Autodesk Inventor part; units mm, degrees
ref_plane "YZ Plane" through (0, 0, 0) normal (1, 0, 0) x (0, 1, 0)
ref_plane "XZ Plane" through (0, 0, 0) normal (0, 1, 0) x (-1, 0, 0)
ref_plane "XY Plane" through (0, 0, 0) normal (0, 0, 1) x (1, 0, 0)
sketch "Sketch1" plane through (0, 0, 0) normal (0, 1, 0) x (-1, 0, 0)
  line L0 (0, 0) -> (20, 0)
  line L1 (0, 0) -> (0, -7.35)
  line L2 (0, -7.35) -> (20, -7.35)
  circle A0 centre (28, -3.675) radius 3
  line L3 (20, -7.35) -> (28, -6.675)
  line L4 (20, 0) -> (28, -0.675)
  dimension "d0" = 20
  dimension "d1" = 7.35
extrude "Extrusion1" add sketch "Sketch1" along normal blind 2
sketch "Sketch3" plane through (0, 2, 0) normal (0, 1, 0) x (1, 0, 0)
  line L0 (0, 0) -> (0, 7.35)
  line L1 (-4.5, 2.25) -> (-14, 2.25)
  line L2 (0, 0) -> (0, 3.68)
  line L3 (0, 0) -> (0, 5.1)
  line L4 (-4.5, 5.1) -> (-14, 5.1)
  line L5 (0, 7.35) -> (-20, 7.35)
  line L6 (-20, 0) -> (0, 0)
  arc A0 (-14, 5.1) -> (-14, 2.25) centre (-14, 3.675) ccw
  arc A1 (-4.5, 2.25) -> (-4.5, 5.1) centre (-4.525, 3.675) ccw
extrude "Extrusion3" cut sketch "Sketch3" against normal blind 10
sketch "Sketch4" plane through (0, 2, 0) normal (0, 1, 0) x (1, 0, 0)
  line L0 (0, 0) -> (-28, 0)
  line L1 (-20, 0) -> (0, 0)
  arc A0 (-28, 6.675) -> (-28, 0.675) centre (-28, 3.675) ccw
  line L2 (-28, 0) -> (-28, 6.675)
  dimension "d20" = 28
extrude "Extrusion4" cut sketch "Sketch4" against normal blind 10
sketch "Sketch5" plane through (0, 2, 0) normal (0, 1, 0) x (1, 0, 0)
  line L0 (-28, 0.675) -> (-20, 0)
  line L1 (-20, 0) -> (-20, 7.35)
  line L2 (-20, 7.35) -> (-28, 6.675)
  line L3 (-20, 7.35) -> (-28, 6.675)
  line L4 (-28, 6.675) -> (-28, 0.675)
  line L5 (-28, 0.675) -> (-20, 0)
  point P0 (0, 0)
extrude "Extrusion5" cut sketch "Sketch5" against normal blind 10
sketch "Sketch7" plane through (0, 2, 0) normal (0, 1, 0) x (1, 0, 0)
  line L0 (0, 0) -> (0, 3.675)
  circle A0 centre (-28.5, 3.675) radius 2.5
  line L1 (-20, 0) -> (0, 0)
  line L2 (-20, 0) -> (-28.8358, 1.1977)
  line L3 (0, 7.35) -> (-20, 7.35)
  line L4 (-20, 7.35) -> (-28.8358, 6.1523)
  line L5 (-20, 7.35) -> (-20, 0)
  line L6 (-20, 7.35) -> (-20, 0)
  dimension "d42" = 5
extrude "Extrusion6" add sketch "Sketch7" against normal blind 2
sketch "Sketch8" plane through (0, 2, 0) normal (0, 1, 0) x (1, 0, 0)
  line L0 (0, 0) -> (0, 7.35)
  circle A0 centre (-22, 3.675) radius 0.67
  circle A1 centre (-25, 3.675) radius 0.67
  circle A2 centre (-28, 3.675) radius 0.67
  dimension "d46" = 1.34
  dimension "d48" = 1.34
  dimension "d50" = 1.34
extrude "Extrusion7" cut sketch "Sketch8" against normal blind 2
properties part number "MMAE 232 Assignment 2_Servo Horn 1 - Dylan Tamras"
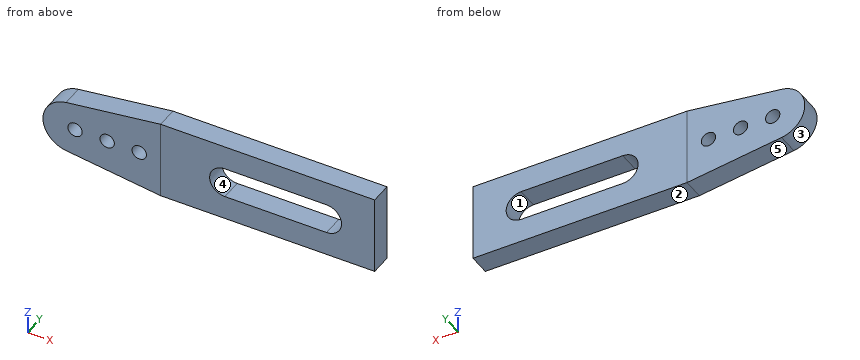
Can you work these out from the model? Positions are in its coordinate system, mm. Face numbers are marked on the shaded views. A direction names the side the tool comes from. Round coordinates to 2 decimals unless told otherwise and drop trailing zeros. Order: outer loops, then holes, each group sorted by start corner. A loop starts at its lowest first (then second) coordinate and runs counter-clockwise, first axis right, second up. Notation, with made-up numbers: (-26.5, 17) -> (-16.5, 17) arc R23 cw to (-16.5, 27) -> close; hole circle Ø2 at (-8.75, 7.25). An arc over 180 degrees is marked (long way). Write each question's results on one line, items separated by ' | '. Start each with the question number.
Item 1: Will this pin go through, and if not, where does the flat tip stop? pin 1 (1.1 mm diameter, centred on x = -25, z = -3.675, fed in from +Y).
Item 2: Which directions (+Z, -Z, +X, -X, +Y, -Y) give clear straight access to the entire face, cutting with the end or side of a thin tool? Please do the marked faces 4 and 5.
Item 3: Please list where these lines run through material, in increasing order: L1, parallel to Z at x = -11.5, y = 1.7; L2, parallel to Z at x = -28, y = 0.1 (3 decimals); L3, parallel to X at y = 0.25, z = -3.5.
Item 4: If we section it at C-C, the plane z = -4: Write out the boundary of the cut face in (x, y), then the cut area to 3 significant figures.
Item 5: If we section it at B-B, the plane y = 1.1: Write out the boundary of the cut face in (x, z) (3 decimals), then the cut area to 3 significant figures.
Item 6: If we section it at A-A, the plane x = -13.5: Write out the boundary of the cut face in (y, z), then the cut area to 3 significant figures.
Item 7: If we section it at D-D, the plane x = -25: Write out the boundary of the cut face in (y, z) (3 decimals), then the cut area to 3 significant figures.
Item 8: Thinking about a two-plate mould opening in X: for the marked faces 1, 2 and 3, which applies, +X half, -X half, draft (parallel to the pull), parting line (faces both ways), or undercut?
Results:
1) pin 1: passes through
2) face 4: +Y, -Y | face 5: -Z, -X, +Y, -Y
3) L1: z = -7.35 to -5.1, -2.25 to 0 | L2: z = -6.266 to -4.345, -3.005 to -1.084 | L3: x = -30.99 to -28.65, -27.35 to -25.65, -24.35 to -22.65, -21.35 to -15.41, -3.11 to 0
4) outline: (-30.98, 0) -> (-28.59, 0) -> (-28.59, 2) -> (-30.98, 2) -> close; (-27.41, 0) -> (-25.59, 0) -> (-25.59, 2) -> (-27.41, 2) -> close; (-24.41, 0) -> (-22.59, 0) -> (-22.59, 2) -> (-24.41, 2) -> close; (-21.41, 0) -> (-15.39, 0) -> (-15.39, 2) -> (-21.41, 2) -> close; (-3.14, 0) -> (0, 0) -> (0, 2) -> (-3.14, 2) -> close | area: 30.4 mm2
5) outline: (-28.836, -6.152) -> (-20, -7.35) -> (0, -7.35) -> (0, 0) -> (-20, 0) -> (-28.836, -1.198) arc R2.5 ccw to start; hole circle Ø1.34 at (-28, -3.675); hole circle Ø1.34 at (-25, -3.675); hole circle Ø1.34 at (-22, -3.675); hole (-14, -5.1) -> (-4.5, -5.1) arc R1.425 ccw to (-4.5, -2.25) -> (-14, -2.25) arc R1.425 ccw to start | area: 172 mm2
6) outline: (0, -7.35) -> (2, -7.35) -> (2, -5.1) -> (0, -5.1) -> close; (0, -2.25) -> (2, -2.25) -> (2, 0) -> (0, 0) -> close | area: 9.00 mm2
7) outline: (0, -6.672) -> (2, -6.672) -> (2, -4.345) -> (0, -4.345) -> close; (0, -3.005) -> (2, -3.005) -> (2, -0.678) -> (0, -0.678) -> close | area: 9.31 mm2
8) face 1: undercut | face 2: draft | face 3: -X half
